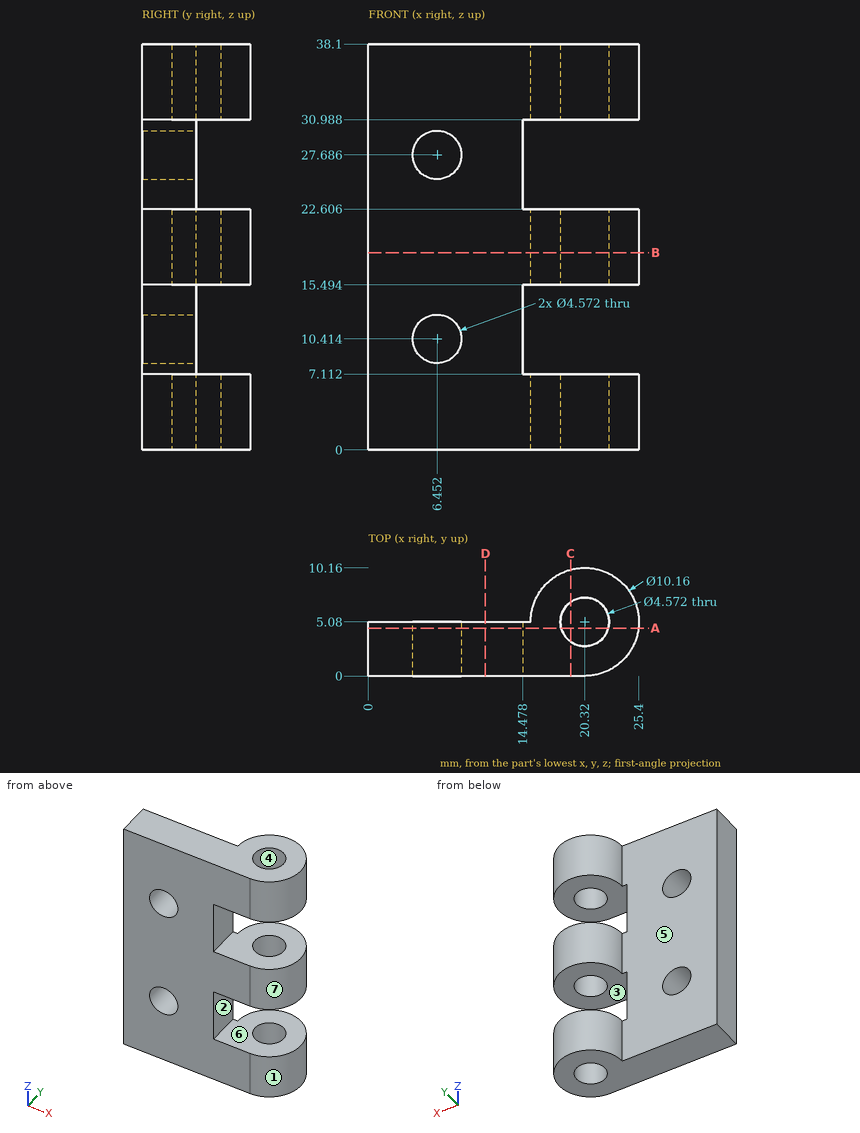
Study the drawing (mm; zero at the part's minimum x, y, z) and answer. A direction names the side the tool comes from. Give positions to 0.01 mm unless a question says otherwise; leave off trailing zeros. Write each loop counter-clockwise with the first axis right and the second up, starting at its lowest first coordinate (ties: lowest second). Pieces come first, ordered by that corner, then holes.
(1) Flat-ended cylindrical pins translate along their axes: pin 1 Ø6 at (y, z) = (8.5, 21) entering from -X; pin 2 Ø2.5 at (x, y) = (20.32, 5.08) entering from -Z; pin 3 Ø5 at (x, y) = (22, 6) entering from -Z; pin 4 Ø1.5 at (y, z) = (2.5, 13) entering from +X. Find the tip coordinate at first contact, or state that the pin passes through.
Final values:
pin 1: stops at x = 15.26
pin 2: passes through
pin 3: stops at z = 0
pin 4: stops at x = 14.48
(2) The part is cut by section A-A on y = 4.5. Write down the section's boundary in (x, z), plus the area to 3 significant figures.
Final values:
outline: (0, 0) - (18.11, 0) - (18.11, 7.11) - (14.48, 7.11) - (14.48, 15.49) - (18.11, 15.49) - (18.11, 22.61) - (14.48, 22.61) - (14.48, 30.99) - (18.11, 30.99) - (18.11, 38.1) - (0, 38.1) - close; (22.53, 0) - (25.37, 0) - (25.37, 7.11) - (22.53, 7.11) - close; (22.53, 15.49) - (25.37, 15.49) - (25.37, 22.61) - (22.53, 22.61) - close; (22.53, 30.99) - (25.37, 30.99) - (25.37, 38.1) - (22.53, 38.1) - close; hole circle Ø4.57 at (6.45, 10.41); hole circle Ø4.57 at (6.45, 27.69)
area: 657 mm2
(3) The part is cut by section C-C on x = 19. Write down the section's boundary in (y, z) (1 decimal).
Final values:
outline: (0, 0) - (3.2, 0) - (3.2, 7.1) - (0, 7.1) - close; (0, 15.5) - (3.2, 15.5) - (3.2, 22.6) - (0, 22.6) - close; (0, 31) - (3.2, 31) - (3.2, 38.1) - (0, 38.1) - close; (6.9, 0) - (10, 0) - (10, 7.1) - (6.9, 7.1) - close; (6.9, 15.5) - (10, 15.5) - (10, 22.6) - (6.9, 22.6) - close; (6.9, 31) - (10, 31) - (10, 38.1) - (6.9, 38.1) - close
(4) The mould has two halves that part along X. Classify the marked faces 1, 2, 3 and 4: pulls with the +X half, pulls with the -X half, needs draft (parallel to the pull), parting line crosses it, or undercut.
Final values:
face 1: parting line crosses it
face 2: pulls with the +X half
face 3: needs draft
face 4: undercut
(5) The part is cut by section D-D on x = 11. Write down the section's boundary in (y, z).
Final values:
outline: (0, 0) - (5.08, 0) - (5.08, 38.1) - (0, 38.1) - close
(6) Which of the six approach directions +Z, -Z, +X, -X, +Y, -Y give full straight-line access (tool end or side, diameter ignored) to the marked faces 5, 6 and 7?
Final values:
face 5: +Z, -Z, -X, +Y
face 6: +X, +Y, -Y
face 7: +Z, -Z
(7) The part is cut by section B-B on z = 18.5. Write down the section's boundary in (x, y), plus the area to 3 significant figures.
Final values:
outline: (0, 0) - (20.32, 0) arc R5.08 ccw (long way) to (15.24, 5.08) - (0, 5.08) - close; hole circle Ø4.57 at (20.32, 5.08)
area: 148 mm2
(8) Straight lines are drawn through the part: line 1 (Z direction, x = 23, y = 1.5); line 2 (Y direction, x = 20.32, z = 18.25); line 3 (X direction, y = 5.25, z = 3). For each, find the intervals that lie inside material, in ascending order.
Final values:
line 1: z = 0 to 7.11, 15.49 to 22.61, 30.99 to 38.1
line 2: y = 0 to 2.79, 7.37 to 10.16
line 3: x = 15.24 to 18.04, 22.6 to 25.4
